The model under review builds one solid part; all positions refer to its coordinate system, in mm. Face numbers are marked on the shaded views. A direction names the side the tool comes from. Round coordinates to 2 decimals unless told otherwise and drop trailing zeros. Loops run counter-clockwise (first coordinate to the right, second up) from the corner with the lowest first, then second, coordinate; pieces in that order, holes last. Notation, with made-up numbers: M 66,-19.5 L 93,-19.5 A8 cw 93,-5.5 Z; hole C 41,9.25 d9. An arc over 180 degrees is marked long. Answer as a JSON object with one key per item and string values. Group by question number.
Item 1: To check wall thickness, follow line 1 (Y direction, x = -13.5, z = 0.5); line 2 (Y direction, x = -15, z = 22.5); line 3 (X direction, y = -7.5, z = 4.25). State the ranges of each line that lie inside material, in increasing order.
Item 2: Consider section B-B (y = 41.5). Give the boundary of the cut face in (x, z).
Item 3: Insertion check: P1, Ø3, axis at x = 22, y = -30.5, coming from the -Z side; P2, Ø3, axis at x = -4, y = 35, coming from the -Z side; P3, Ø4.5, axis at x = -26, y = -40, coming from the -Z side. Each pin has a flat end and moves straight along its axis. Give the tip position at first contact, or say it passes through.
Item 4: Tool access review of the marked faces 1, 2 and 3: name each direction out of +Z, -Z, +X, -X, +Y, -Y from which nothing blocks a thin tool from reaching the whole face with its end or side.
Item 5: Consider section A-A (z = 11.75). Give the boundary of the cut face in (x, y).
Item 6: Consider section D-D (x = -5). Give the boundary of the cut face in (y, z).
Item 7: The part is to be moulded in two halves that separate along X. For the marked faces 4, 5, 6 and 7, say which applies: +X half, -X half, draft (parallel to the pull), parting line (faces both ways), or undercut.
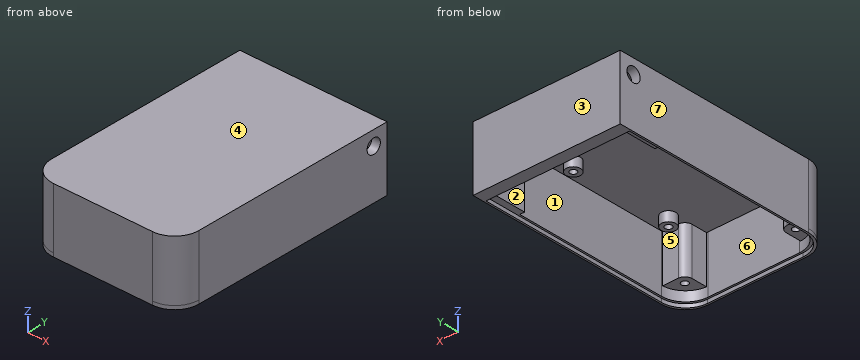
```python
from build123d import *

# Parameters (mm, degrees)
SKETCH1_W               = 61
SKETCH1_H               = 95
BOSS_EXTRUDE1_DEPTH     = 25
SHELL1_T                = -1.5
FILLET1_R               = 10
SKETCH2_R               = 3
SKETCH2_R_2             = 1.4
BOSS_EXTRUDE2_DEPTH     = 4
SKETCH4_W               = 2
SKETCH4_H               = 18
BOSS_EXTRUDE3_DEPTH     = 23.5
SKETCH3_R               = 3
CUT_EXTRUDE1_DEPTH      = 1
CUT_EXTRUDE1_DEPTH_BACK = 62
BOSS_EXTRUDE4_DEPTH     = 1.5
SKETCH6_W               = 59.5
SKETCH6_H               = 4.25
BOSS_EXTRUDE5_DEPTH     = 1.5
SKETCH7_W               = 52
SKETCH7_H               = 1
BOSS_EXTRUDE6_DEPTH     = 1
FILLET2_R               = 0.3
BOSS_EXTRUDE7_DEPTH     = 19.5
SKETCH9_R               = 1.4
CUT_EXTRUDE2_DEPTH      = 10


with BuildPart() as part:
    # Sketch1 → Boss-Extrude1 (new body)
    with BuildSketch(Plane.XY):
        Rectangle(SKETCH1_W, SKETCH1_H)
    extrude(amount=BOSS_EXTRUDE1_DEPTH)

    # Shell1
    shell1_openings = [part.faces().sort_by_distance(p)[0] for p in [
        (0, 0, 0),
    ]]
    offset(amount=SHELL1_T, openings=shell1_openings, kind=Kind.INTERSECTION)

    # Fillet1
    fillet1_edges = [part.edges().sort_by_distance(p)[0] for p in [
        (29, -46, 11.75),
        (-29, -46, 11.75),
        (30.5, -47.5, 12.5),
        (-30.5, -47.5, 12.5),
    ]]
    fillet(fillet1_edges, radius=FILLET1_R)

    # Sketch2 → Boss-Extrude2 (add)
    with BuildSketch(Plane(origin=(0, 0, 23.5), x_dir=(-1, 0, 0), z_dir=(0, 0, -1))):
        with Locations((-21.5, 12)):
            Circle(SKETCH2_R)
        with Locations((-21.5, 12)):
            Circle(SKETCH2_R_2, mode=Mode.SUBTRACT)
        with Locations((-21.5, -31)):
            Circle(SKETCH2_R)
        with Locations((-21.5, -31)):
            Circle(SKETCH2_R_2, mode=Mode.SUBTRACT)
        with Locations((21.5, -31)):
            Circle(SKETCH2_R)
        with Locations((21.5, -31)):
            Circle(SKETCH2_R_2, mode=Mode.SUBTRACT)
    extrude(amount=BOSS_EXTRUDE2_DEPTH)

    # Sketch4 → Boss-Extrude3 (add)
    with BuildSketch(Plane(origin=(0, 0, 23.5), x_dir=(-1, 0, 0), z_dir=(0, 0, -1))):
        with Locations((-28, 37)):
            Rectangle(SKETCH4_W, SKETCH4_H)
        with Locations((28, 37)):
            Rectangle(SKETCH4_W, SKETCH4_H)
    extrude(amount=BOSS_EXTRUDE3_DEPTH)

    # Sketch3 → Cut-Extrude1 (cut, two sides)
    with BuildSketch(Plane(origin=(30.5, 0, 0), x_dir=(0, 0, -1), z_dir=(1, 0, 0))) as cut_extrude1_sk:
        with Locations((-19, 41.5)):
            Circle(SKETCH3_R)
    extrude(amount=CUT_EXTRUDE1_DEPTH, mode=Mode.SUBTRACT)
    extrude(cut_extrude1_sk.sketch, amount=-CUT_EXTRUDE1_DEPTH_BACK, mode=Mode.SUBTRACT)

    # Sketch5 → Boss-Extrude4 (add)
    with BuildSketch(Plane(origin=(0, 0, 0), x_dir=(-1, 0, 0), z_dir=(0, 0, -1))):
        with BuildLine():
            Line((-30.5, 47.5), (30.5, 47.5))
            Line((30.5, 47.5), (30.5, -37.5))
            ThreePointArc((30.5, -37.5), (27.571067812, -44.571067812), (20.5, -47.5))
            Line((20.5, -47.5), (-20.5, -47.5))
            ThreePointArc((-20.5, -47.5), (-27.571067812, -44.571067812), (-30.5, -37.5))
            Line((-30.5, -37.5), (-30.5, 47.5))
        make_face()
        with BuildLine():
            Line((-19.75, -46.75), (19.75, -46.75))
            ThreePointArc((19.75, -46.75), (26.821067812, -43.821067812), (29.75, -36.75))
            Line((29.75, -36.75), (29.75, 46.75))
            Line((29.75, 46.75), (-29.75, 46.75))
            Line((-29.75, 46.75), (-29.75, -36.75))
            ThreePointArc((-29.75, -36.75), (-26.821067812, -43.821067812), (-19.75, -46.75))
        make_face(mode=Mode.SUBTRACT)
    extrude(amount=BOSS_EXTRUDE4_DEPTH)

    # Sketch6 → Boss-Extrude5 (add)
    with BuildSketch(Plane(origin=(0, 0, 0), x_dir=(-1, 0, 0), z_dir=(0, 0, -1))):
        with Locations((0, 44.625)):
            Rectangle(SKETCH6_W, SKETCH6_H)
    extrude(amount=BOSS_EXTRUDE5_DEPTH)

    # Sketch7 → Boss-Extrude6 (add)
    with BuildSketch(Plane.XY):
        with Locations((0, 43)):
            Rectangle(SKETCH7_W, SKETCH7_H)
    extrude(amount=BOSS_EXTRUDE6_DEPTH)

    # Fillet2
    fillet2_edges = [part.edges().sort_by_distance(p)[0] for p in [
        (0, 43.5, 1),
        (0, 42.5, 1),
    ]]
    fillet(fillet2_edges, radius=FILLET2_R)

    # Sketch8 → Boss-Extrude7 (add)
    with BuildSketch(Plane(origin=(0, 0, 23.5), x_dir=(-1, 0, 0), z_dir=(0, 0, -1))):
        with BuildLine():
            Line((-22.5, -36.5), (-28.987492178, -36.5))
            Line((-28.987492178, -36.5), (-28.987492178, -39))
            ThreePointArc((-28.987492178, -39), (-26.937239646, -43.949747468), (-21.987492178, -46))
            Line((-21.987492178, -46), (-19.5, -46))
            Line((-19.5, -46), (-19.5, -39.5))
            ThreePointArc((-19.5, -39.5), (-20.378679656, -37.378679656), (-22.5, -36.5))
        make_face()
        with BuildLine():
            Line((19.5, -46), (19.5, -39.5))
            ThreePointArc((19.5, -39.5), (20.378679656, -37.378679656), (22.5, -36.5))
            Line((22.5, -36.5), (28.987492178, -36.5))
            Line((28.987492178, -36.5), (28.987492178, -39))
            ThreePointArc((28.987492178, -39), (26.937239646, -43.949747468), (21.987492178, -46))
            Line((21.987492178, -46), (19.5, -46))
        make_face()
    extrude(amount=BOSS_EXTRUDE7_DEPTH)

    # Sketch9 → Cut-Extrude2 (cut)
    with BuildSketch(Plane(origin=(0, 0, 4), x_dir=(-1, 0, 0), z_dir=(0, 0, -1))):
        with Locations((-23, -40)):
            Circle(SKETCH9_R)
        with Locations((23, -40)):
            Circle(SKETCH9_R)
    extrude(amount=-CUT_EXTRUDE2_DEPTH, mode=Mode.SUBTRACT)


solid = part.part
```
Geometry results:
{
 "1": {"line 1": "y = -47.5 to -46, 42.5 to 43.5, 46 to 47.5", "line 2": "y = -47.5 to -46, 46 to 47.5", "line 3": "x = -30.5 to -29, 29 to 30.5"},
 "2": {"outline": "M -30.5,-1.5 L -29.75,-1.5 L -29.75,0 L -27,0 L -27,16 L -30.5,16 Z; M -30.5,22 L -27,22 L -27,23.5 L 27,23.5 L 27,22 L 30.5,22 L 30.5,25 L -30.5,25 Z; M 27,0 L 29.75,0 L 29.75,-1.5 L 30.5,-1.5 L 30.5,16 L 27,16 Z"},
 "3": {"P1": "stops at z = 19.5", "P2": "stops at z = 23.5", "P3": "stops at z = 0"},
 "4": {"face 1": "-Z", "face 2": "none", "face 3": "+Z, -Z, +X, -X, +Y"},
 "5": {"outline": "M -30.5,-37.5 A10 ccw -20.5,-47.5 L 20.5,-47.5 A10 ccw 30.5,-37.5 L 30.5,47.5 L -30.5,47.5 Z; hole M -29,-36 A10 ccw -28.99,-36.5 L -22.5,-36.5 A3 cw -19.5,-39.5 L -19.5,-45.99 A10 ccw -19,-46 L 19,-46 A10 ccw 19.5,-45.99 L 19.5,-39.5 A3 cw 22.5,-36.5 L 28.99,-36.5 A10 ccw 29,-36 L 29,28 L 27,28 L 27,46 L -27,46 L -27,28 L -29,28 Z; hole C -23,-40 d2.8; hole C 23,-40 d2.8"},
 "6": {"outline": "M -47.5,-1.5 L -46.75,-1.5 L -46.75,0 L -46,0 L -46,23.5 L 46,23.5 L 46,0 L 43.5,0 L 43.5,0.7 A0.3 ccw 43.2,1 L 42.8,1 A0.3 ccw 42.5,0.7 L 42.5,-1.5 L 47.5,-1.5 L 47.5,25 L -47.5,25 Z"},
 "7": {"face 4": "draft", "face 5": "undercut", "face 6": "undercut", "face 7": "-X half"}
}
